Check sheet for the drawn part. Datum: minimum x, y, z corner. Units: mm. Round coordinates to 2 decimals unless told otherwise and drop trailing zeros. Order: outer loops, then holes, each group sorted by start corner. A loop starts at its lowest first (then second) coordinate and runs counter-clockwise, first axis right, second up. Notation, with made-up numbers: (74, 50.5) - (117, 50.5) arc R16 ccw to (117, 78.5) - close; hole circle Ø8 at (-2, 2.25). An arc over 180 degrees is marked (long way). Write each question's results on one line, items separated by ' | '.
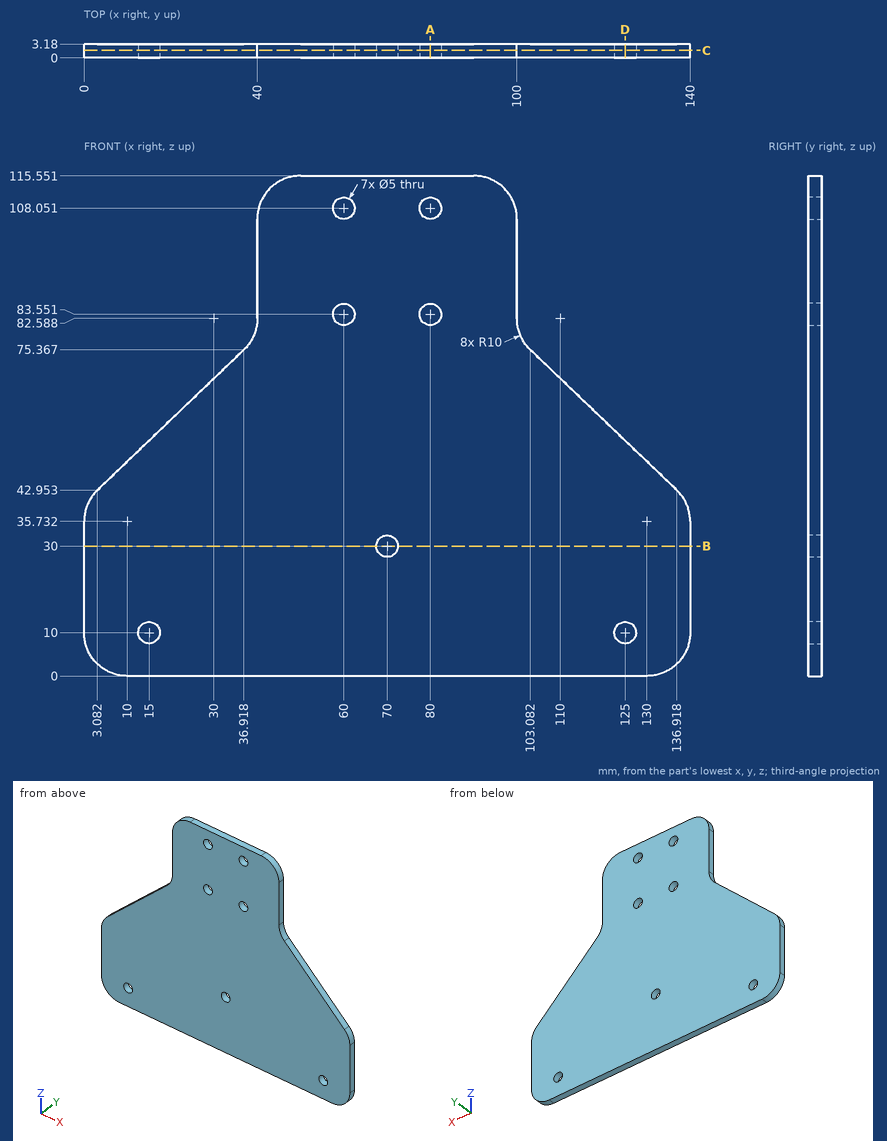
(1) Depth check by flat-ended pin: pin 1 Ø1 at (x, y) = (22.5, 1) entering from +Z (1 decimal); pin 2 Ø1 at (y, z) = (2, 95) entering from +X; pin 3 Ø1.5 at (y, z) = (1, 43.5) entering from +X. Enter the tip coordinate at first touch or a pass-through.
Answers follow:
pin 1: z = 62 | pin 2: x = 100 | pin 3: x = 137.12
(2) Section check C-C (y = 1.7). Record the cut outline in (x, z).
Answers follow:
outline: (0, 10) arc R10 ccw to (10, 0) - (130, 0) arc R10 ccw to (140, 10) - (140, 35.73) arc R10 ccw to (136.92, 42.95) - (103.08, 75.37) arc R10 cw to (100, 82.59) - (100, 105.55) arc R10 ccw to (90, 115.55) - (50, 115.55) arc R10 ccw to (40, 105.55) - (40, 82.59) arc R10 cw to (36.92, 75.37) - (3.08, 42.95) arc R10 ccw to (0, 35.73) - close; hole circle Ø5 at (15, 10); hole circle Ø5 at (60, 83.55); hole circle Ø5 at (60, 108.05); hole circle Ø5 at (70, 30); hole circle Ø5 at (80, 83.55); hole circle Ø5 at (80, 108.05); hole circle Ø5 at (125, 10)
(3) Section check A-A (x = 80). Record the cut outline in (y, z).
Answers follow:
outline: (0, 0) - (3.18, 0) - (3.18, 81.05) - (0, 81.05) - close; (0, 86.05) - (3.18, 86.05) - (3.18, 105.55) - (0, 105.55) - close; (0, 110.55) - (3.18, 110.55) - (3.18, 115.55) - (0, 115.55) - close
(4) Material ranges on line 1 (Z direction, x = 80, y = 2.2); line 2 (X direction, y = 0.95, z = 10); line 3 (Z direction, x = 70, y = 1.7), recorded low to high.
Answers follow:
line 1: 0 to 81.05, 86.05 to 105.55, 110.55 to 115.55 | line 2: 0 to 12.5, 17.5 to 122.5, 127.5 to 140 | line 3: 0 to 27.5, 32.5 to 115.55
(5) Section check B-B (z = 30). Record the cut outline in (x, y).
Answers follow:
outline: (0, 0) - (67.5, 0) - (67.5, 3.18) - (0, 3.18) - close; (72.5, 0) - (140, 0) - (140, 3.18) - (72.5, 3.18) - close
(6) Section check D-D (x = 125). Record the cut outline in (y, z).
Answers follow:
outline: (0, 0) - (3.18, 0) - (3.18, 7.5) - (0, 7.5) - close; (0, 12.5) - (3.18, 12.5) - (3.18, 54.37) - (0, 54.37) - close
